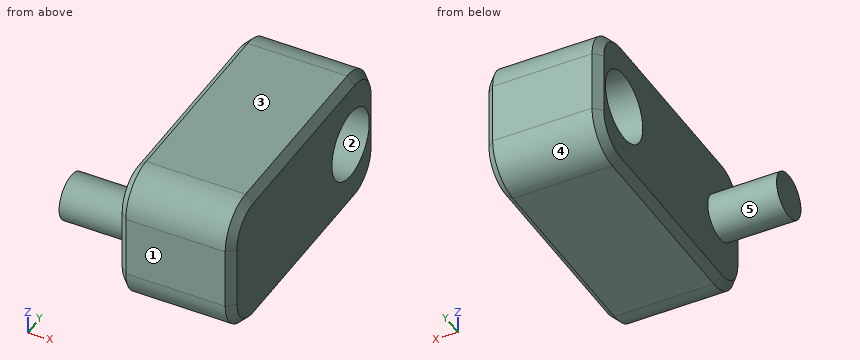
```python
from build123d import *

# Parameters (mm, degrees)
F0_W     = 75
F0_H     = 90
F1_DEPTH = 175
F2_R     = 25
F3_SIZE  = 5
F4_R     = 23
F5_DEPTH = 75.001
F6_R     = 15
F7_DEPTH = 45


with BuildPart() as f1:
    # F0 (on Front) → F1 (new body)
    with BuildSketch(Plane.XZ):
        Rectangle(F0_W, F0_H)
    extrude(amount=F1_DEPTH)

    # F2
    f2_edges = [f1.edges().sort_by_distance(p)[0] for p in [
        (0, 0, 45),
        (0, 0, -45),
        (0, -175, -45),
        (0, -175, 45),
    ]]
    fillet(f2_edges, radius=F2_R)

    # F3
    f3_edges = [f1.edges().sort_by_distance(p)[0] for p in [
        (-37.5, -87.5, 45),
        (37.5, -167.67767, 37.67767),
    ]]
    chamfer(f3_edges, length=F3_SIZE)

    # F4 (on face) → F5 (cut, through all)
    with BuildSketch(Plane(origin=(-37.5, 0, 0), x_dir=(0, -1, 0), z_dir=(-1, 0, 0))):
        with Locations((30, 0)):
            Circle(F4_R)
    extrude(amount=-F5_DEPTH, mode=Mode.SUBTRACT)

    # F6 (on face) → F7 (join)
    with BuildSketch(Plane(origin=(-37.5, 0, 0), x_dir=(0, -1, 0), z_dir=(-1, 0, 0))):
        with Locations((148, 0)):
            Circle(F6_R)
    extrude(amount=F7_DEPTH)


solid = f1.part
```
The model under review builds one solid part; all positions refer to its coordinate system, in mm. Face numbers are marked on the shaded views. A direction names the side the tool comes from. Give positions to 0.01 mm unless a question says otherwise; leave off trailing zeros. Write each loop counter-clockwise with the first axis right and the second up, starting at its lowest first coordinate (ties: lowest second). Pieces come first, ordered by that corner, then holes.
(1) Tool access review of the marked faces 4 and 5: name each direction out of +Z, -Z, +X, -X, +Y, -Y from which nothing blocks a thin tool from reaching the whole face with its end or side.
(2) Consider section C-C, the plane x = -18. Give the boundary of the cut face in (y, z), and give its area (3 significant figures).
(3) To check wall thickness, follow L1, parallel to Z at x = 12.5, y = -30; L2, parallel to Y at x = 28, z = -0.5; L3, parallel to X at y = -115.5, z = 23. State the ranges of each line that lie inside material, in increasing order.
(4) The part is to be moulded in two halves that separate along Z. For the marked faces 1, 2 and 3, say which applies: released by +Z, released by -Z, zero draft, split by the parting line, or undercut.
(5) Consider section B-B, the plane z = 0. Give the boundary of the cut face in (x, y).
(6) Consider section D-D, the plane y = -136. Give the boundary of the cut face in (x, z).
(7) Consider section A-A, the plane y = -30. Give the boundary of the cut face in (x, z).
(8) For P1, Ø4, axis at y = -64.5, z = -20, coming from the -X side; P2, Ø4, axis at x = 8.5, z = 24.5, coming from the +Y side; P3, Ø24, axis at y = -127, z = 15.5, coming from the -X side, all flat-tipped, find the tip position at first contact; note any pin that passes through.
Returned:
1. face 4: -Z, +X, -X, +Y
1. face 5: -X
2. outline: (-175, -20) arc R25 ccw to (-150, -45) - (-25, -45) arc R25 ccw to (0, -20) - (0, 20) arc R25 ccw to (-25, 45) - (-150, 45) arc R25 ccw to (-175, 20) - close; hole circle Ø46 at (-30, 0)
2. area: 13,600 mm2
3. L1: z = -45 to -23, 23 to 45
3. L2: y = -175 to -52.99, -7.01 to 0
3. L3: x = -37.5 to 37.5
4. face 1: zero draft
4. face 2: undercut
4. face 3: released by +Z
5. outline: (-82.5, -163) - (-37.5, -163) - (-37.5, -170) - (-32.5, -175) - (32.5, -175) - (37.5, -170) - (37.5, -53) - (-37.5, -53) - (-37.5, -133) - (-82.5, -133) - close; (-37.5, -7) - (37.5, -7) - (37.5, -5) - (32.5, 0) - (-32.5, 0) - (-37.5, -5) - close
6. outline: (-82.5, -9) - (-37.5, -9) - (-37.5, -40) - (-32.5, -45) - (32.5, -45) - (37.5, -40) - (37.5, 40) - (32.5, 45) - (-32.5, 45) - (-37.5, 40) - (-37.5, 9) - (-82.5, 9) - close
7. outline: (-37.5, -40) - (-32.5, -45) - (32.5, -45) - (37.5, -40) - (37.5, -23) - (-37.5, -23) - close; (-37.5, 23) - (37.5, 23) - (37.5, 40) - (32.5, 45) - (-32.5, 45) - (-37.5, 40) - close
8. P1: stops at x = -37.5
8. P2: stops at y = -0.13
8. P3: stops at x = -82.5
